```python
from build123d import *

# Parameters (mm, degrees)
SKETCH1_W           = 5.54
SKETCH1_H           = 6.3
BOSS_EXTRUDE1_DEPTH = 8.8
SKETCH2_W           = 0.8
SKETCH2_H           = 0.5
BOSS_EXTRUDE2_DEPTH = 3.6
CUT_EXTRUDE1_REACH  = 7.54
SKETCH4_W           = 2
SKETCH4_H           = 4
CUT_EXTRUDE2_DEPTH  = 3.15
CUT_EXTRUDE2_TAPER  = 10


with BuildPart() as part:
    # Sketch1 → Boss-Extrude1 (new body)
    with BuildSketch(Plane(origin=(0, 0, 0), x_dir=(1, 0, 0), z_dir=(0, 1, 0))):
        Rectangle(SKETCH1_W, SKETCH1_H)
    extrude(amount=BOSS_EXTRUDE1_DEPTH)

    # Sketch2 → Boss-Extrude2 (add)
    with BuildSketch(Plane(origin=(0, 0, 0), x_dir=(1, 0, 0), z_dir=(0, 1, 0))):
        with Locations((1.27, 0.2)):
            Rectangle(SKETCH2_W, SKETCH2_H)
        with Locations((-1.27, 0.2)):
            Rectangle(SKETCH2_W, SKETCH2_H)
    extrude(amount=-BOSS_EXTRUDE2_DEPTH)

    # Sketch3 → Cut-Extrude1 (cut, up to next)
    with BuildSketch(Plane(origin=(2.77, 0, 0), x_dir=(0, 0, -1), z_dir=(1, 0, 0)), mode=Mode.PRIVATE) as cut_extrude1_sk1:
        with BuildLine():
            ThreePointArc((-3.15, 4.7), (-2.974264069, 5.124264069), (-2.55, 5.3))
            Line((-2.55, 5.3), (-2.337822174, 5.3))
            Line((-2.337822174, 5.3), (-1.4, 8.8))
            Line((-1.4, 8.8), (-3.15, 8.8))
            Line((-3.15, 8.8), (-3.15, 4.7))
        make_face()
    cut_extrude1_tool1 = extrude(cut_extrude1_sk1.sketch, amount=-CUT_EXTRUDE1_REACH, mode=Mode.PRIVATE) & part.part
    add(cut_extrude1_tool1.solids().sort_by_distance((2.77, 7.227986, 2.489914))[0], mode=Mode.SUBTRACT)
    # Sketch3 → Cut-Extrude1 (cut, up to next)
    with BuildSketch(Plane(origin=(2.77, 0, 0), x_dir=(0, 0, -1), z_dir=(1, 0, 0)), mode=Mode.PRIVATE) as cut_extrude1_sk2:
        Polygon((3.15, 8.8), (1.4, 8.8), (3.15, 2.268911087), align=None)
    cut_extrude1_tool2 = extrude(cut_extrude1_sk2.sketch, amount=-CUT_EXTRUDE1_REACH, mode=Mode.PRIVATE) & part.part
    add(cut_extrude1_tool2.solids().sort_by_distance((2.77, 6.62297, -2.566667))[0], mode=Mode.SUBTRACT)

    # Sketch4 → Cut-Extrude2 (cut)
    with BuildSketch(Plane.XY.offset(3.15)):
        with Locations((-1.27, 2.268911087)):
            Rectangle(SKETCH4_W, SKETCH4_H)
        with Locations((1.27, 2.268911087)):
            Rectangle(SKETCH4_W, SKETCH4_H)
    extrude(amount=-CUT_EXTRUDE2_DEPTH, taper=CUT_EXTRUDE2_TAPER, mode=Mode.SUBTRACT)


solid = part.part
```
Design review of the part built by this model. Coordinates are the model's own, in mm. A direction names the side the tool comes from. Give positions to 0.01 mm unless a question says otherwise; leave off trailing zeros. Loops run counter-clockwise (first coordinate to the right, second up) from the corner with the lowest first, then second, coordinate; pieces in that order, holes last. Notation, with made-up numbers: (-23, -0.5) -> (-8, -0.5) arc R20 ccw to (-8, 30.5) -> close; hole circle Ø1 at (-11, 32). An arc over 180 degrees is marked (long way). Write each question's results on one line, items separated by ' | '.
Q1. Take a section at C-C, the plane z = 2.75. Give the number of separate pieces and of enclosed holes in the cut face, plus the area to 3 significant figures.
Reply:
separate pieces: 1 | enclosed holes: 2 | area: 14.8 mm²
Q2. Machinability: for faces 4 (the face through (1, 2, 0)), 5 (the face through (0.039, 7.026, 1.875)), which of the approach directions +Z, -Z, +X, -X, +Y, -Y give a long, thin tool a straight path to every point of the face, cutting with its end or side? Answer none if there is none.
Reply:
face 4: +Z | face 5: +Z, +X, -X, +Y
Q3. Take a section at A-A, the plane y = -2. Write out the cut boundary in (x, z), plus the area to 3 significant figures.
Reply:
outline: (-1.67, -0.45) -> (-0.87, -0.45) -> (-0.87, 0.05) -> (-1.67, 0.05) -> close; (0.87, -0.45) -> (1.67, -0.45) -> (1.67, 0.05) -> (0.87, 0.05) -> close | area: 0.800 mm²
Q4. Take a section at D-D, the plane y = 8.25. Write out the cut boundary in (x, z).
Reply:
outline: (-2.77, -1.55) -> (2.77, -1.55) -> (2.77, 1.55) -> (-2.77, 1.55) -> close
Q5. Take a section at B-B, the plane x = 0.15. Write out the cut boundary in (y, z).
Reply:
outline: (0, -3.15) -> (2.27, -3.15) -> (8.8, -1.4) -> (8.8, 1.4) -> (5.3, 2.34) -> (5.3, 2.55) arc R0.6 ccw to (4.7, 3.15) -> (0, 3.15) -> close
Q6. The part is to be moulded in two halves that separate along Y. For faces 1 (the face through (0, 1, -3.15)), 2 (the face through (0, 8.8, 0)), 3 (the face through (-1, 2, 0)), say which applies: +Y half, -Y half, draft (parallel to the pull), parting line (faces both ways), or undercut.
Reply:
face 1: draft | face 2: +Y half | face 3: undercut
Q7. For pin 1 Ø0.9 at (x, y) = (1.5, -2) entering from +Z; pin 2 Ø0.6 at (y, z) = (-1.5, 0) entering from +X, all flat-tipped, find the tip position at first contact; note any pin that passes through.
Reply:
pin 1: stops at z = 0.05 | pin 2: stops at x = 1.67
Q8. Wall thickness on L1, parallel to X at y = 3.25, z = 0.5; L2, parallel to Y at x = -2.25, z = 2.5; L3, parallel to Y at x = 0.05, z = -1.25: over which ranges is each line inside the solid? List them lowest first.
Reply:
L1: x = -2.77 to -1.8, -0.74 to 0.74, 1.8 to 2.77 | L2: y = 0 to 5.3 | L3: y = 0 to 8.8
